Here's how the part is built. I have some questions about the finished solid (model axes, mm). A direction names the side the tool comes from. Give positions to 0.01 mm unless a question says otherwise; leave off trailing zeros. Order: outer loops, then holes, each group sorted by start corner. A loop starts at its lowest first (then second) coordinate and runs counter-clockwise, first axis right, second up.
from build123d import *

# Parameters (mm, degrees)
SKETCH1_W           = 31.62
SKETCH1_H           = 17
BOSS_EXTRUDE1_DEPTH = 17
SKETCH2_W           = 27.32
SKETCH2_H           = 6.7
BOSS_EXTRUDE2_DEPTH = 9.7
SKETCH3_W           = 31.62
SKETCH3_H           = 5
BOSS_EXTRUDE3_DEPTH = 32.7
SKETCH4_R           = 2
SKETCH4_R_2         = 4.75
CUT_EXTRUDE1_DEPTH  = 5
FILLET1_R           = 10
FILLET2_R           = 5


with BuildPart() as part:
    # Sketch1 → Boss-Extrude1 (new body)
    with BuildSketch(Plane(origin=(0, 0, 0), x_dir=(1, 0, 0), z_dir=(0, 1, 0))):
        Rectangle(SKETCH1_W, SKETCH1_H)
    extrude(amount=BOSS_EXTRUDE1_DEPTH)

    # Sketch2 → Boss-Extrude2 (add)
    with BuildSketch(Plane(origin=(0, 0, -8.5), x_dir=(-1, 0, 0), z_dir=(0, 0, -1))):
        with Locations((0, 8.5)):
            Rectangle(SKETCH2_W, SKETCH2_H)
    extrude(amount=BOSS_EXTRUDE2_DEPTH)

    # Sketch3 → Boss-Extrude3 (add)
    with BuildSketch(Plane(origin=(0, 17, 0), x_dir=(1, 0, 0), z_dir=(0, 1, 0))):
        with Locations((0, -6)):
            Rectangle(SKETCH3_W, SKETCH3_H)
    extrude(amount=BOSS_EXTRUDE3_DEPTH)

    # Sketch4 → Cut-Extrude1 (cut)
    with BuildSketch(Plane.XY.offset(8.5)):
        with Locations((0, 29.025)):
            Circle(SKETCH4_R)
        with Locations((-10.28, 37.5)):
            Circle(SKETCH4_R)
        with Locations((0, 45.975)):
            Circle(SKETCH4_R)
        with Locations(Location((10.28, 37.5, 0), (0, 0, 180))):
            Circle(SKETCH4_R)
        with Locations((0, 37.5)):
            Circle(SKETCH4_R_2)
    extrude(amount=-CUT_EXTRUDE1_DEPTH, mode=Mode.SUBTRACT)

    # Fillet1
    fillet1_edges = [part.edges().sort_by_distance(p)[0] for p in [
        (15.81, 49.7, 6),
        (-15.81, 49.7, 6),
    ]]
    fillet(fillet1_edges, radius=FILLET1_R)

    # Fillet2
    fillet2_edges = [part.edges().sort_by_distance(p)[0] for p in [
        (0, 17, 3.5),
    ]]
    fillet(fillet2_edges, radius=FILLET2_R)


solid = part.part
Q1. For faces 4 (the face through (-0.2, 32.6, 3.5)), 5 (the face through (13.66, 8, -13)), 6 (the face through (0, 5.15, -13)), which set-ups out of +Z, -Z, +X, -X, +Y, -Y let a thin tool reach every point of the face, with its end or its side?
Filled sheet:
face 4: -Z, +X, -X, +Y
face 5: -Z, +X, +Y, -Y
face 6: -Z, +X, -X, -Y
Q2. I'm going to push flat-ended pins straight in: P1, Ø6.5, axis at x = 0, y = 45.975, coming from the -Z side; P2, Ø5, axis at x = -3.5, z = -13, coming from the +Y side; P3, Ø1, axis at x = 12.5, z = -11.5, coming from the -Y side. Where does each tip first touch, or does it pass through?
Filled sheet:
P1: stops at z = 3.5
P2: stops at y = 11.85
P3: stops at y = 5.15
Q3. I need wall thicknesses on L1, parallel to Y at x = 0, z = 7.05 (3 decimals); L2, parallel to Y at x = -8, z = -7.5; L3, parallel to Z at x = -13, y = 30. Which ranges of each line are inside material? Lowest first, please.
Filled sheet:
L1: y = 0 to 27.025, 31.025 to 32.75, 42.25 to 43.975, 47.975 to 49.7
L2: y = 0 to 17
L3: z = 3.5 to 8.5
Q4. If we section it at A-A on x = 0: List the corners of the cut face in (y, z) for me (3 decimals), plus the area to 3 significant figures.
Filled sheet:
outline: (0, -8.5) - (5.15, -8.5) - (5.15, -18.2) - (11.85, -18.2) - (11.85, -8.5) - (17, -8.5) - (17, -1.5) arc R5 cw to (22, 3.5) - (27.025, 3.5) - (27.025, 8.5) - (0, 8.5) - close; (31.025, 3.5) - (32.75, 3.5) - (32.75, 8.5) - (31.025, 8.5) - close; (42.25, 3.5) - (43.975, 3.5) - (43.975, 8.5) - (42.25, 8.5) - close; (47.975, 3.5) - (49.7, 3.5) - (49.7, 8.5) - (47.975, 8.5) - close
area: 435 mm2
Q5. If we section it at B-B on y = 37.5: List the corners of the cut face in (x, z) for me.
Filled sheet:
outline: (-15.81, 3.5) - (-12.28, 3.5) - (-12.28, 8.5) - (-15.81, 8.5) - close; (-8.28, 3.5) - (-4.75, 3.5) - (-4.75, 8.5) - (-8.28, 8.5) - close; (4.75, 3.5) - (8.28, 3.5) - (8.28, 8.5) - (4.75, 8.5) - close; (12.28, 3.5) - (15.81, 3.5) - (15.81, 8.5) - (12.28, 8.5) - close
Q6. If we section it at D-D on z = 6.75: List the corners of the cut face in (x, y) for me (3 decimals).
Filled sheet:
outline: (-15.81, 0) - (15.81, 0) - (15.81, 39.7) arc R10 ccw to (5.81, 49.7) - (-5.81, 49.7) arc R10 ccw to (-15.81, 39.7) - close; hole circle Ø4 at (-10.28, 37.5); hole circle Ø9.5 at (0, 37.5); hole circle Ø4 at (0, 29.025); hole circle Ø4 at (0, 45.975); hole circle Ø4 at (10.28, 37.5)
Q7. If we section it at C-C on x = -10.28: List the corners of the cut face in (y, z) for me, plus the area to 3 significant figures.
Filled sheet:
outline: (0, -8.5) - (5.15, -8.5) - (5.15, -18.2) - (11.85, -18.2) - (11.85, -8.5) - (17, -8.5) - (17, -1.5) arc R5 cw to (22, 3.5) - (35.5, 3.5) - (35.5, 8.5) - (0, 8.5) - close; (39.5, 3.5) - (48.65, 3.5) - (48.65, 8.5) - (39.5, 8.5) - close
area: 498 mm2
Q8. Thinking about a two-plate mould opening in Y: for faces 1 (the face through (-10.714, 35.548, 6.035)), 2 (the face through (0, 49.7, 6)), 3 (the face through (0, 9, -18.2)), which applies, released by +Y, released by -Y, zero draft, split by the parting line, or undercut?
Filled sheet:
face 1: undercut
face 2: released by +Y
face 3: zero draft
